Could you check a few things on this model? Use its own coordinates, in mm. A direction names the side the tool comes from. Give positions to 0.01 mm unless a question says otherwise; leave off trailing zeros. Order: outer loops, then holes, each group sorted by start corner. A loop starts at its lowest first (then second) coordinate and runs counter-clockwise, first axis right, second up. Notation, with made-up numbers: (80.5, -30.75) - (135.5, -30.75) arc R17 ccw to (135.5, -20.75) - close; hole circle Ø8 at (-24, 76.5). An arc over 180 degrees is marked (long way). One line per question, with ' | ' between items. Start each with the question number.
1. I need wall thicknesses on probe 1 along Z at (x, y) = (40, 33); probe 2 along Z at (x, y) = (0, 29); probe 3 along Y at (x, z) = (27.5, -1). Which ranges of each line are inside material? Lowest first, please. Write a range as from..to.
2. If we mould it in two halves opening along Z, with no side actions, what happens to faces 1 (the flat face through (-1, 30, 110)), 2 (the cylindrical face through (-25.015, 29.72, 0.66)), 3 (the flat face through (-1, 0, 34)), 4 (the flat face through (-1, 30, -40))? For each: released by +Z, released by -Z, zero draft, split by the parting line, or undercut.
3. For P1, Ø6, axis at x = 49.5, z = -2, coming from the +Y side; P2, Ø24, axis at x = 2, z = 72, coming from the +Y side; P3, Ø6, axis at x = 53, z = 5, coming from the +Y side, each with a flat end and sliding along its axis, tell me the tip position at first contact or that it passes through.
4. Which directions (+Z, -Z, +X, -X, +Y, -Y) give clear straight access to the entire face, cutting with the end or side of a thin tool? Please do faces 5 (the flat face through (40, 10, 0)), 6 (the flat face through (-75, 30, 34)).
5. Imagine slicing it at D-D (x = 0). Please give me the cut outline in (y, z).
6. Imagine slicing it at C-C (y = 26). Please give me the cut outline in (x, z), and give its area (3 significant figures).
7. Imagine slicing it at A-A (z = 0). Please give me the cut outline in (x, y).
8. Imagine slicing it at B-B (x = 40). Please give me the cut outline in (y, z), and give its area (3 significant figures).
```python
from build123d import *

# Parameters (mm, degrees)
SKETCH1_W           = 150
SKETCH1_H           = 80
BOSS_EXTRUDE1_DEPTH = 60
SKETCH3_W           = 150
SKETCH3_H           = 60
BOSS_EXTRUDE2_DEPTH = 70


with BuildPart() as part:
    # Sketch1 → Boss-Extrude1 (new body)
    with BuildSketch(Plane(origin=(0, 0, 0), x_dir=(1, 0, 0), z_dir=(0, 1, 0))):
        Rectangle(SKETCH1_W, SKETCH1_H)
    extrude(amount=BOSS_EXTRUDE1_DEPTH)

    # Sketch2 → Cut-Revolve1 (revolve, cut)
    with BuildSketch(Plane.XY):
        Polygon((-40, 60), (-70, 60), (-55, 50), (-55, 10), (-40, 10), align=None)
    cut_revolve1 = revolve(axis=Axis((-40, 10, 0), (0, 1, 0)), mode=Mode.SUBTRACT)

    # Mirror1: Cut-Revolve1 across plane
    add(cut_revolve1.mirror(Plane(origin=(0, 0, 0), x_dir=(0, 0, 1), z_dir=(1, 0, 0))), mode=Mode.SUBTRACT)

    # Sketch3 → Boss-Extrude2 (add)
    with BuildSketch(Plane.XY.offset(40)):
        with Locations((0, 30)):
            Rectangle(SKETCH3_W, SKETCH3_H)
    extrude(amount=BOSS_EXTRUDE2_DEPTH)

    # Sketch6 → Cut-Revolve2 (revolve, cut)
    with BuildSketch(Plane(origin=(0, 0, 0), x_dir=(0, 0, -1), z_dir=(1, 0, 0))):
        Polygon((-64.678891041, 60), (-64.678891041, 10), (-79.678891041, 10), (-79.678891041, 50), (-89.678891041, 60), align=None)
    revolve(axis=Axis((0, 60, 64.678891041), (0, -1, 0)), mode=Mode.SUBTRACT)


solid = part.part
```
Results found:
1) probe 1: z = -40..-15, 15..110 | probe 2: z = -40..49.68, 79.68..110 | probe 3: y = 0..10
2) face 1: released by +Z | face 2: undercut | face 3: zero draft | face 4: released by -Z
3) P1: stops at y = 10 | P2: stops at y = 54.59 | P3: stops at y = 51.29
4) face 5: +Y | face 6: +Z, -Z, -X, +Y, -Y
5) outline: (0, -40) - (60, -40) - (60, 39.68) - (50, 49.68) - (10, 49.68) - (10, 79.68) - (50, 79.68) - (60, 89.68) - (60, 110) - (0, 110) - close
6) outline: (-75, -40) - (75, -40) - (75, 110) - (-75, 110) - close; hole circle Ø30 at (-40, 0); hole circle Ø30 at (0, 64.68); hole circle Ø30 at (40, 0) | area: 20,400 mm2
7) outline: (-75, 0) - (75, 0) - (75, 60) - (70, 60) - (55, 50) - (55, 10) - (25, 10) - (25, 50) - (10, 60) - (-10, 60) - (-25, 50) - (-25, 10) - (-55, 10) - (-55, 50) - (-70, 60) - (-75, 60) - close
8) outline: (0, -40) - (60, -40) - (60, -30) - (50, -15) - (10, -15) - (10, 15) - (50, 15) - (60, 30) - (60, 110) - (0, 110) - close | area: 7,350 mm2
